```python
from build123d import *

# Parameters (mm, degrees)
F0_R     = 10
F1_DEPTH = 14
F4_R     = 8
F5_DEPTH = 12
F6_D     = 7


with BuildPart() as f1:
    # F0 (on Top) → F1 (new body)
    with BuildSketch(Plane.XY):
        Circle(F0_R)
    extrude(amount=F1_DEPTH)

    # F4 (on offset) → F5 (cut)
    with BuildSketch(Plane.XY.offset(14)):
        Circle(F4_R)
    extrude(amount=-F5_DEPTH, mode=Mode.SUBTRACT)

    # F6 (through all)
    with Locations(Plane.XY.offset(14)):
        with Locations((0, 0)):
            Hole(F6_D / 2)


solid = f1.part
```
Build history of the part. All positions in model axes, mm. A direction names the side the tool comes from. Give positions to 0.01 mm unless a question says otherwise; leave off trailing zeros. Loops run counter-clockwise (first coordinate to the right, second up) from the corner with the lowest first, then second, coordinate; pieces in that order, holes last. Notation, with made-up numbers: (22.25, 10) -> (55.25, 10) arc R13 ccw to (55.25, 23) -> close; hole circle Ø4 at (-19, 30). An arc over 180 degrees is marked (long way). One line per question, with ' | ' between items. Start each with the question number.
1) Two-plate mould, pull along Y, no slides. Class faces 1 (the flat face through (0, 8.2, 14)), 2 (the cylindrical face through (-3.233, -1.341, 0.986)), 3 (the cylindrical face through (-2.17, -9.76, 6.9)): released by +Y, released by -Y, zero draft, split by the parting line, or undercut.
2) 3-axis set-ups, long thin cutter, end or side, ignore diameter. For faces 4 (the cylindrical face through (-1.73, -7.81, 8.08)), 5 (the flat face through (0, -4, 0)): which of +Z, -Z, +X, -X, +Y, -Y reach the whole face in a straight line?
3) Cut at C-C (z = 3.75). Give the cut face in (x, y).
4) Pin check, flat tips, straight feed: pin 1 (4 mm diameter, centred on x = 0, y = 0, fed in from +Z); pin 2 (6 mm diameter, centred on y = 7.5, z = 5, fed in from +X); pin 3 (1 mm diameter, centred on x = -5, y = 3.5, fed in from +Z); pin 4 (8 mm diameter, centred on x = 7, z = 12.5, fed in from -Y). Stop position of each tip, or through.
5) Cut at D-D (x = 7.25). Give the cut face in (y, z).
6) Cut at A-A (x = 0). Give the cut face in (y, z), plus the area to 3 significant figures.
7) Probe L1, parallel to Y at x = 0, z = 8.5; L2, parallel to Y at x = 0, z = 1; L3, parallel to Z at x = 6.25, y = 1. List the from-to ranges inside material, lowest first.
Return value:
1) face 1: zero draft | face 2: undercut | face 3: split by the parting line
2) face 4: +Z | face 5: -Z, +X, -X, +Y, -Y
3) outline: circle Ø20 at (0, 0); hole circle Ø16 at (0, 0)
4) pin 1: through | pin 2: x = 8.93 | pin 3: z = 2 | pin 4: y = -9.54
5) outline: (-6.89, 0) -> (6.89, 0) -> (6.89, 14) -> (3.38, 14) -> (3.38, 2) -> (-3.38, 2) -> (-3.38, 14) -> (-6.89, 14) -> close
6) outline: (-10, 0) -> (-3.5, 0) -> (-3.5, 2) -> (-8, 2) -> (-8, 14) -> (-10, 14) -> close; (3.5, 0) -> (10, 0) -> (10, 14) -> (8, 14) -> (8, 2) -> (3.5, 2) -> close | area: 74.0 mm^2
7) L1: -10 to -8, 8 to 10 | L2: -10 to -3.5, 3.5 to 10 | L3: 0 to 2
